from build123d import *

# Parameters (mm, degrees)
F1_DEPTH = 10
F2_R     = 2
F3_DEPTH = 25
F4_R     = 1.5
F5_DEPTH = 4


with BuildPart() as f1:
    # F0 (on Front) → F1 (new body)
    with BuildSketch(Plane.XZ):
        Polygon((-13, 0), (0, 0), (0, 21), (-3, 21), (-3, 3), (-13, 3), align=None)
    extrude(amount=F1_DEPTH)

    # F2 (on face) → F3 (cut)
    with BuildSketch(Plane(origin=(-3, 0, 0), x_dir=(0, -1, 0), z_dir=(-1, 0, 0))):
        with Locations((5, 18)):
            Circle(F2_R)
        with Locations((5, 10)):
            Circle(F2_R)
    extrude(amount=-F3_DEPTH, mode=Mode.SUBTRACT)

    # F4 (on face) → F5 (join)
    with BuildSketch(Plane.XY.offset(3)):
        with Locations((-10, -5)):
            Circle(F4_R)
    extrude(amount=F5_DEPTH)


solid = f1.part
Verification items for the finished model (mm, model axes). A direction names the side the tool comes from. Coordinates: 2 decimals unless noted, no trailing zeros. Order: outer loops, then holes, each group sorted by start corner. A loop starts at its lowest first (then second) coordinate and runs counter-clockwise, first axis right, second up. Notation, with made-up numbers: M -26.75,-21 L 8.25,-21 A12 cw 8.25,-3 Z; hole C 61.25,27.25 d1. An arc over 180 degrees is marked long. One line per item, written item: value. Start each with the question number.
Item 1: Sectioned sample at C-C on x = -10. Record the cut outline in (y, z).
Item 2: Thickness scan on probe 1 along Z at (x, y) = (-1.2, -5); probe 2 along Z at (x, y) = (-3.75, -6.5); probe 3 along X at (y, z) = (-3, 17.5). Record the ranges inside material, lowest first.
Item 3: Access from +Z, -Z, +X, -X, +Y, -Y to the whole of each face (thin tool, end or side, straight path). Record for faces 1 (the flat face through (-8, -5, 3)), 2 (the flat face through (-10, -5, 7)), 3 (the flat face through (-2.7, 0, 7.4)).
Item 4: Sectioned sample at D-D on y = -2. Record the cut outline in (x, z), then the cut area to 3 significant figures.
Item 5: Sectioned sample at B-B on z = 18. Record the cut outline in (x, y).
Item 6: Sectioned sample at A-A on y = -5. Record the cut outline in (x, z).
Item 7: Depth check by flat-ended pin: P1, Ø1.5, axis at x = -9.5, y = -5.5, coming from the +Z side; P2, Ø5, axis at x = -8.5, z = 7, coming from the -Y side. Enter the tip coordinate at first touch or a pass-through.
Item 8: Mould release check, pull along X, two halves, no side actions. Record for faces 4 (the flat face through (0, -4, 8)), 5 (the cylindrical face through (-11.5, -4.93, 4.97)), 6 (the flat face through (-1, -5, 21)): pulls with the +X half, pulls with the -X half, needs draft (parallel to the pull), parting line crosses it, or undercut.
Calculated:
1. outline: M -10,0 L 0,0 L 0,3 L -3.5,3 L -3.5,7 L -6.5,7 L -6.5,3 L -10,3 Z
2. probe 1: 0 to 8, 12 to 16, 20 to 21
2. probe 2: 0 to 3
2. probe 3: -3 to 0
3. face 1: +Z
3. face 2: +Z, -X, +Y, -Y
3. face 3: +Z, -Z, +X, -X, +Y
4. outline: M -13,0 L 0,0 L 0,21 L -3,21 L -3,3 L -13,3 Z
4. area: 93.0 mm^2
5. outline: M -3,-10 L 0,-10 L 0,-7 L -3,-7 Z; M -3,-3 L 0,-3 L 0,0 L -3,0 Z
6. outline: M -13,0 L 0,0 L 0,8 L -3,8 L -3,3 L -8.5,3 L -8.5,7 L -11.5,7 L -11.5,3 L -13,3 Z; M -3,12 L 0,12 L 0,16 L -3,16 Z; M -3,20 L 0,20 L 0,21 L -3,21 Z
7. P1: z = 7
7. P2: y = -6.5
8. face 4: pulls with the +X half
8. face 5: undercut
8. face 6: needs draft
